The figure shows three views and two pictorial views of one solid part (mm, origin at its lowest corner). Answer the questions. A direction names the side the tool comes from. Coordinates: 2 decimals unless noted, no trailing zeros. Order: outer loops, then holes, each group sorted by start corner. A loop starts at its lowest first (then second) coordinate and runs counter-clockwise, first axis right, second up. Notation, with made-up numbers: (86.5, 37.25) -> (121.5, 37.25) arc R22 ccw to (121.5, 55.25) -> close; hole circle Ø7 at (52, 55). An arc over 180 degrees is marked (long way). Return JSON: item names as keys, results as strings.
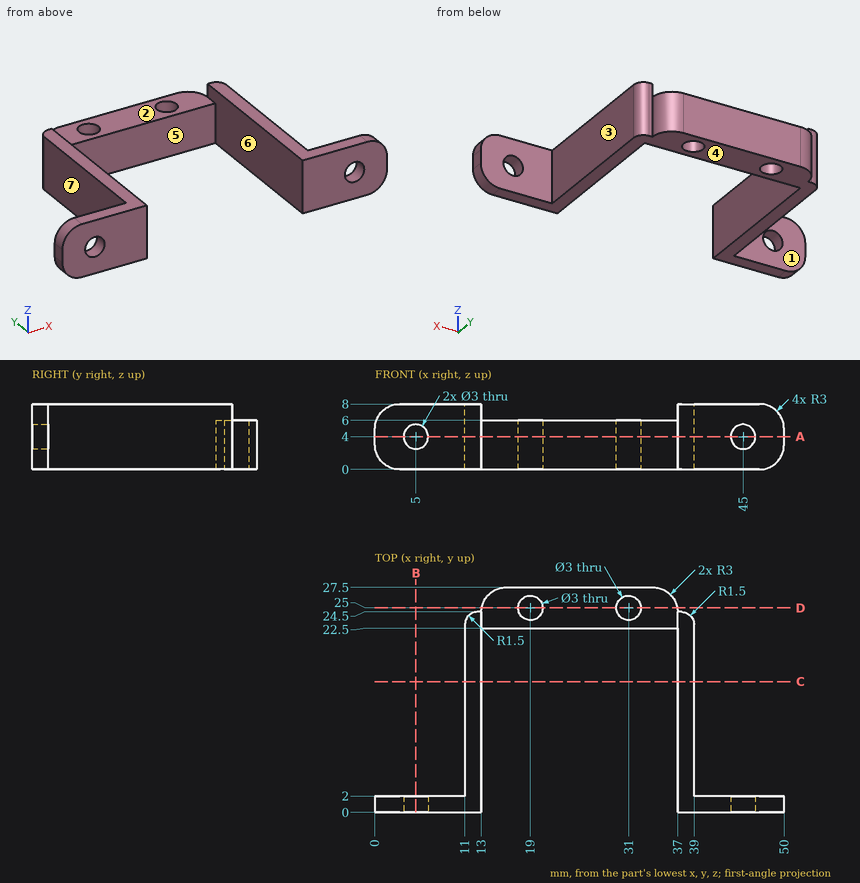
Item 1: Determine the mould class of the marked faces 4, 5, 6 and 7 for opening direction X: pulls with the +X half, pulls with the -X half, needs draft (parallel to the pull), parting line crosses it, or undercut.
Answer list:
{"face 4": "needs draft", "face 5": "undercut", "face 6": "undercut", "face 7": "pulls with the -X half"}
Item 2: The part is cut by section C-C on y = 16. Determine the outline of the cut face in (x, z).
Answer list:
{"outline": "(11, 0) -> (13, 0) -> (13, 8) -> (11, 8) -> close; (37, 0) -> (39, 0) -> (39, 8) -> (37, 8) -> close"}
Item 3: The part is cut by section D-D on y = 25. Determine the outline of the cut face in (x, z), plus the area to 4 significant figures.
Answer list:
{"outline": "(13.04, 0) -> (17.5, 0) -> (17.5, 6) -> (13.04, 6) -> close; (20.5, 0) -> (29.5, 0) -> (29.5, 6) -> (20.5, 6) -> close; (32.5, 0) -> (36.96, 0) -> (36.96, 6) -> (32.5, 6) -> close", "area": "107.5 mm2"}
Item 4: Which of the six approach directions +Z, -Z, +X, -X, +Y, -Y give full straight-line access (tool end or side, diameter ignored) to the marked faces 1, 2 and 3?
Answer list:
{"face 1": "+Z, -Z, -X, +Y", "face 2": "+Z, +Y, -Y", "face 3": "+Z, -Z, +X, +Y"}
Item 5: The part is cut by section B-B on x = 5. Determine the outline of the cut face in (y, z), plus the area to 3 significant figures.
Answer list:
{"outline": "(0, 0) -> (2, 0) -> (2, 2.5) -> (0, 2.5) -> close; (0, 5.5) -> (2, 5.5) -> (2, 8) -> (0, 8) -> close", "area": "10.0 mm2"}
Item 6: Flat-ended cylindrical pins translate along their axes: pin 1 (3 mm diameter, centred on x = 16, y = 17, fed in from +Z); pin 2 (2.5 mm diameter, centred on x = 25, y = 26, fed in from +Z); pin 3 (4 mm diameter, centred on y = 12.5, z = 5, fed in from +X); pin 4 (2 mm diameter, centred on x = 31, z = 3.5, fed in from -Y). Find the tip coordinate at first contact, or state that the pin passes through.
Answer list:
{"pin 1": "through", "pin 2": "z = 6", "pin 3": "x = 39", "pin 4": "y = 22.5"}
Item 7: The part is cut by section A-A on z = 4. Count the separate pieces of the cut face and the enclosed holes in it, plus the area to 3 significant figures.
Answer list:
{"separate pieces": "3", "enclosed holes": "2", "area": "231 mm2"}
Item 8: Find the intervals of material crossed by probe 1 along X at (y, z) = (1.6, 4); probe 2 along X at (y, z) = (9.75, 0.75); probe 3 along Y at (x, z) = (31, 3.8), in increasing order.
Answer list:
{"probe 1": "0 to 3.5, 6.5 to 13, 37 to 43.5, 46.5 to 50", "probe 2": "11 to 13, 37 to 39", "probe 3": "22.5 to 23.5, 26.5 to 27.5"}
